Check sheet for the modelled part. Datum: model origin and axes. Units: mm. Coordinates: 2 decimals unless noted, no trailing zeros. Loops run counter-clockwise (first coordinate to the right, second up) from the corner with the lowest first, then second, coordinate; pieces in that order, holes last. Notation, with made-up numbers: (-22.75, -14) - (-2.75, -14) arc R29 ccw to (-2.75, 23) - close; hole circle Ø2 at (15.25, 20.25). An arc over 180 degrees is marked (long way). Use a Markdown table: item, result. Add a question column.
1) Sectioned sample at A-A, the plane x = 0.5. Enter the section's corners in (y, z).
2) Go/stop test with flat-tipped pins: P1, Ø5, axis at x = -10.5, y = 4.5, coming from the -Z side; P2, Ø6, axis at x = 17, y = 2.5, coming from the +Z side; P3, Ø12, axis at x = 3, y = 13, coming from the +Z side. Record where each tip stops, or that it passes through.
3) Thickness scan on line 1 (Y direction, x = -19, z = 0.2); line 2 (Y direction, x = -42, z = 1.85); line 3 (Y direction, x = -19.5, z = 1.2). Record the ranges inside material, lowest first.
4) Sectioned sample at B-B, the plane z = 1.7. Enter the section's corners in (x, y), then the cut area to 3 significant figures.
5) Draft check along Y on faces 1 (the flat face through (-36.98, 16.99, 1.29)), 2 (the flat face through (-37, 16.01, 1.23)), 3 (the flat face through (-9, 2, 0)), 4 (the cylindrical face through (-0.533, -1.878, 2.508)). Enter one of: pulls with the +Y half, pulls with the -Y half, needs draft (parallel to the pull), parting line crosses it, or undercut.
from build123d import *

# Parameters (mm, degrees)
F1_DEPTH    = 5.08
F0_W        = 76.2
F0_H        = 5.08
F2_DEPTH    = 5.08
F3_T1_DEPTH = 88.9
F3_T4_ANGLE = 251.0303843405
F3_T6_ANGLE = 292.9828431402


# Not quite as in the source:
# - a fillet or chamfer that OpenCascade refuses, or shapes differently, is made with other operations: its cross-section is extruded or revolved along the edge and cut away or added


with BuildPart() as f1:
    # F0 (on Top) → F1 (new body)
    with BuildSketch(Plane.XY):
        with BuildLine():
            Line((-38.1, -2.54), (-38.1, 2.54))
            ThreePointArc((-38.1, 2.54), (-44.5507724238, 8.9907724238), (-38.1, 15.4415448477))
            Line((-38.1, 15.4415448477), (-36.2862832844, 16.3751454373))
            Line((-36.2862832844, 16.3751454373), (-38.1, 17.9815448477))
            ThreePointArc((-38.1, 17.9815448477), (-48.3607724238, 7.7207724238), (-38.1, -2.54))
        make_face()
    extrude(amount=F1_DEPTH)

    # F0 (on Top) → F2 (join)
    with BuildSketch(Plane.XY):
        Rectangle(F0_W, F0_H)
    extrude(amount=F2_DEPTH)

    # F3: fillet of radius 5.08 on 2 edges, made by hand

    # F3_s2 → F3_t1 (cut)
    with BuildSketch(Plane.YZ.offset(-38.1)):
        with BuildLine():
            ThreePointArc((-2.54, 5.08), (1.0521024484, 3.5921024484), (2.54, 0))
            Line((2.54, 0), (2.54, 5.08))
            Line((2.54, 5.08), (-2.54, 5.08))
        make_face()
        with BuildLine():
            ThreePointArc((-2.54, 0), (-1.0521024484, 3.5921024484), (2.54, 5.08))
            Line((2.54, 5.08), (-2.54, 5.08))
            Line((-2.54, 5.08), (-2.54, 0))
        make_face()
    extrude(amount=F3_T1_DEPTH, mode=Mode.SUBTRACT)

    # F3_s3 → F3_t4 (revolve, cut)
    with BuildSketch(Plane(origin=(-6.3994276616, 18.6173540989, 0), x_dir=(0, 0, 1), z_dir=(0.3250666938, -0.9456910936, 0))):
        with BuildLine():
            ThreePointArc((0, 23.2602922785), (3.5921024484, 24.7481898301), (5.08, 28.3402922785))
            Line((5.08, 28.3402922785), (5.08, 23.2602922785))
            Line((5.08, 23.2602922785), (0, 23.2602922785))
        make_face()
    revolve(axis=Axis((-38.1, 7.7207724238, 5.08), (0, 0, 1)), revolution_arc=F3_T4_ANGLE, mode=Mode.SUBTRACT)

    # F3_s5 → F3_t6 (revolve, cut)
    with BuildSketch(Plane.YZ.offset(-38.1)):
        with BuildLine():
            ThreePointArc((-2.54, 5.08), (1.0521024484, 3.5921024484), (2.54, 0))
            Line((2.54, 0), (2.54, 5.08))
            Line((2.54, 5.08), (-2.54, 5.08))
        make_face()
    revolve(axis=Axis((-38.1, 8.9907724238, 5.08), (0, 0, -1)), revolution_arc=F3_T6_ANGLE, mode=Mode.SUBTRACT)


solid = f1.part
Solved:
| question | item | result |
|---|---|---|
| 1 | outline | (-2.54, 0) - (2.54, 0) arc R5.08 ccw to (0, 4.4) arc R5.08 ccw to start |
| 2 | P1 | stops at z = 0 |
| 2 | P2 | stops at z = 4.4 |
| 2 | P3 | passes through |
| 3 | line 1 | y = -2.54 to 2.54 |
| 3 | line 2 | y = -1.39 to 3.42, 14.56 to 16.83 |
| 3 | line 3 | y = -2.4 to 2.4 |
| 4 | outline | (-38.1, -2.25) - (38.1, -2.25) - (38.1, 2.25) - (-38.1, 2.25) arc R6.74 cw (long way) to (-37.57, 15.71) - (-36.29, 16.38) - (-37.76, 17.68) arc R9.97 ccw (long way) to start |
| 4 | area | 429 mm2 |
| 5 | face 1 | pulls with the +Y half |
| 5 | face 2 | undercut |
| 5 | face 3 | needs draft |
| 5 | face 4 | pulls with the -Y half |
